```python
from build123d import *

# Parameters (mm, degrees)
EXTRUDE_RAIL_PROFILE_DEPTH     = 125
CBORE_FOR_M3_SHCS2_D           = 3.5
CBORE_FOR_M3_SHCS2_CBORE_D     = 6
CBORE_FOR_M3_SHCS2_CBORE_DEPTH = 4
FILL_START                     = -0.75
FILL_PATTERN_OUTLINE_R         = 3
FILL_PATTERN_DEPTH             = 4
FILL_START_2                   = -3.25
FILL_PATTERN_2_OUTLINE_R       = 1.75
FILL_PATTERN_2_DEPTH           = 2.5


# Read off the part's stored shape, not the designer's step: Fill Pattern
with BuildPart() as part:
    # Sketch1 → Extrude Rail Profile (new body)
    with BuildSketch(Plane.XY):
        with BuildLine():
            Line((-4.3, -3.25), (4.3, -3.25))
            Line((4.3, -3.25), (4.5, -3.05))
            Line((4.5, -3.05), (4.5, 0.455012563))
            ThreePointArc((4.5, 0.455012563), (3.924845827, 0.712323349), (3.617735397, 1.2625))
            Line((3.617735397, 1.2625), (3.15008224, 1.2625))
            Line((3.15008224, 1.2625), (3.15008224, 1.7625))
            Line((3.15008224, 1.7625), (3.65008224, 1.7625))
            ThreePointArc((3.65008224, 1.7625), (3.973877727, 2.229724887), (4.5, 2.444987437))
            Line((4.5, 2.444987437), (4.5, 3.05))
            Line((4.5, 3.05), (4.3, 3.25))
            Line((4.3, 3.25), (-4.3, 3.25))
            Line((-4.3, 3.25), (-4.5, 3.05))
            Line((-4.5, 3.05), (-4.5, 2.444987437))
            ThreePointArc((-4.5, 2.444987437), (-3.973877727, 2.229724887), (-3.65008224, 1.7625))
            Line((-3.65008224, 1.7625), (-3.15008224, 1.7625))
            Line((-3.15008224, 1.7625), (-3.15008224, 1.2625))
            Line((-3.15008224, 1.2625), (-3.617735397, 1.2625))
            ThreePointArc((-3.617735397, 1.2625), (-3.924845827, 0.712323349), (-4.5, 0.455012563))
            Line((-4.5, 0.455012563), (-4.5, -3.05))
            Line((-4.5, -3.05), (-4.3, -3.25))
        make_face()
    extrude(amount=EXTRUDE_RAIL_PROFILE_DEPTH)

    # CBORE for M3 SHCS2 (through all)
    with Locations(Plane(origin=(0, 3.25, 0), x_dir=(1, 0, 0), z_dir=(0, 1, 0))):
        with Locations((0, -10)):
            cbore_for_m3_shcs2 = CounterBoreHole(CBORE_FOR_M3_SHCS2_D / 2, CBORE_FOR_M3_SHCS2_CBORE_D / 2, CBORE_FOR_M3_SHCS2_CBORE_DEPTH)

    # Mirror 2: CBORE for M3 SHCS2 across plane
    add(cbore_for_m3_shcs2.mirror(Plane.XY.offset(62.5)), mode=Mode.SUBTRACT)

    # Fill Pattern outline → Fill Pattern (cut)
    with BuildSketch(Plane(origin=(0, 0, 0), x_dir=(1, 0, 0), z_dir=(0, 1, 0)).offset(FILL_START)):
        with Locations((0, -30)):
            Circle(FILL_PATTERN_OUTLINE_R)
        with Locations((0, -50)):
            Circle(FILL_PATTERN_OUTLINE_R)
        with Locations((0, -70)):
            Circle(FILL_PATTERN_OUTLINE_R)
        with Locations((0, -90)):
            Circle(FILL_PATTERN_OUTLINE_R)
    extrude(amount=FILL_PATTERN_DEPTH, mode=Mode.SUBTRACT)

    # Fill Pattern 2 outline → Fill Pattern 2 (cut)
    with BuildSketch(Plane(origin=(0, 0, 0), x_dir=(1, 0, 0), z_dir=(0, 1, 0)).offset(FILL_START_2)):
        with Locations((0, -30)):
            Circle(FILL_PATTERN_2_OUTLINE_R)
        with Locations((0, -50)):
            Circle(FILL_PATTERN_2_OUTLINE_R)
        with Locations((0, -70)):
            Circle(FILL_PATTERN_2_OUTLINE_R)
        with Locations((0, -90)):
            Circle(FILL_PATTERN_2_OUTLINE_R)
    extrude(amount=FILL_PATTERN_2_DEPTH, mode=Mode.SUBTRACT)


solid = part.part
```
Design review of the part built by this model. Coordinates are the model's own, in mm. A direction names the side the tool comes from. Coordinates: 2 decimals unless noted, no trailing zeros. Order: outer loops, then holes, each group sorted by start corner. A loop starts at its lowest first (then second) coordinate and runs counter-clockwise, first axis right, second up. Notation, with made-up numbers: M 36,67 L 94,67 A15 cw 94,87 Z; hole C -32,-1.75 d11. An arc over 180 degrees is marked long. Answer as a JSON object with one key per item and string values. Group by question number.
1) Mouldability with a two-part tool opening along X and no side actions: class faces 3 (the flat face through (0, 0, 0)), 4 (the cylindrical face through (0, 1, 7)), 5 (the flat face through (-4.5, -1, 62)) as pulls with the +X half, pulls with the -X half, needs draft (parallel to the pull), parting line crosses it, or undercut.
2) Tool access review of faces 1 (the cylindrical face through (-0.38, -2.02, 71.71)), 2 (the flat face through (2, -0.75, 90)): name each direction out of +Z, -Z, +X, -X, +Y, -Y from which nothing blocks a thin tool from reaching the whole face with its end or side.
3) Wall thickness on L1, parallel to X at y = 1.3, z = 30; L2, parallel to X at y = -1.6, z = 115; L3, parallel to Y at x = 4.25, z = 46.5: over which ranges is each line inside the solid? List them lowest first.
4) For pin 1 (3 mm diameter, centred on x = 0, z = 30, fed in from -Y); pin 2 (3 mm diameter, centred on x = 0.5, z = 69.5, fed in from +Y), all flat-tipped, find the tip position at first contact; note any pin that passes through.
5) Add section C-C, the plane x = 0. Count the separate pieces of the cut face and the enclosed holes in it, then the cut area to 3 significant figures.
6) Add section B-B, the plane z = 55.5. Write out the cut boundary in (x, y), then the cut area to 3 significant figures.
7) Add section A-A, the plane z = 115. Write out the cut boundary in (x, y), then the cut area to 3 significant figures.
Computed values:
{
 "1": {"face 3": "needs draft", "face 4": "undercut", "face 5": "pulls with the -X half"},
 "2": {"face 1": "+Y, -Y", "face 2": "+Y"},
 "3": {"L1": "x = -3.15 to -3, 3 to 3.15", "L2": "x = -4.5 to -1.75, 1.75 to 4.5", "L3": "y = -3.25 to 0.51, 2.39 to 3.25"},
 "4": {"pin 1": "passes through", "pin 2": "stops at y = -0.75"},
 "5": {"separate pieces": "7", "enclosed holes": "0", "area": "616 mm^2"},
 "6": {"outline": "M -4.5,-3.05 L -4.3,-3.25 L 4.3,-3.25 L 4.5,-3.05 L 4.5,0.46 A1 cw 3.62,1.26 L 3.15,1.26 L 3.15,1.76 L 3.65,1.76 A1 cw 4.5,2.44 L 4.5,3.05 L 4.3,3.25 L -4.3,3.25 L -4.5,3.05 L -4.5,2.44 A1 cw -3.65,1.76 L -3.15,1.76 L -3.15,1.26 L -3.62,1.26 A1 cw -4.5,0.46 Z", "area": "55.2 mm^2"},
 "7": {"outline": "M -4.5,-3.05 L -4.3,-3.25 L -1.75,-3.25 L -1.75,-0.75 L -3,-0.75 L -3,3.25 L -4.3,3.25 L -4.5,3.05 L -4.5,2.44 A1 cw -3.65,1.76 L -3.15,1.76 L -3.15,1.26 L -3.62,1.26 A1 cw -4.5,0.46 Z; M 1.75,-3.25 L 4.3,-3.25 L 4.5,-3.05 L 4.5,0.46 A1 cw 3.62,1.26 L 3.15,1.26 L 3.15,1.76 L 3.65,1.76 A1 cw 4.5,2.44 L 4.5,3.05 L 4.3,3.25 L 3,3.25 L 3,-0.75 L 1.75,-0.75 Z", "area": "22.5 mm^2"}
}
